Job drawing, mm, ordinate dimensions from the low corner. One solid piece. A direction names the side the tool comes from. Round coordinates to 2 decimals unless told otherwise and drop trailing zeros. Write each loop counter-clockwise with the first axis right and the second up, starting at its lowest first coordinate (ties: lowest second). Pieces come first, ordered by that corner, then holes. Notation, with made-up numbers: M 89,-6.75 L 110,-6.75 A35 cw 110,29.25 Z; hole C 16,63 d7. An arc over 180 degrees is marked long. Answer as a JSON object with one key per item and string values. Group by question number.
1. Which spindle directions (+Z, -Z, +X, -X, +Y, -Y) get a long thin tool onto all of the face, cutting with end or side? Do the marked faces 1, 2, 3, 4 and 5. Say none if no direction does.
2. Band-saw the part on D-D, the plane z = 2.5. Write the cut outline in (x, y).
3. Band-saw the part on B-B, the plane x = 10. Write the cut outline in (y, z) (1 decimal), plus the area to 3 significant figures.
4. Drop flat-ended pins along their axis: pin 1 (8 mm diameter, centred on y = 30.5, z = 3.5, fed in from +X); pin 2 (3 mm diameter, centred on x = 12, z = 3.5, fed in from -Y); pin 3 (6.5 mm diameter, centred on x = 18, z = 14.5, fed in from +Y); pin 4 (3 mm diameter, centred on x = 10, y = 10, fed in from +Z). Give the stop position or say it passes through.
5. Two-plate mould, pull along Y, no slides. Class the marked faces 6, 7, 8 and 9: +Y half, -Y half, draft (parallel to the pull), parting line (faces both ways), or undercut.
6. Band-saw the part on C-C, the plane x = 17. Write the cut outline in (y, z).
7. Drill centre lines: line 1 (Y direction, x = 10, z = 16.5) (1 decimal); line 2 (X direction, y = 37, z = 17.25); line 3 (Z direction, x = 16.75, y = 18). Where is each one in solid material? Low to high. Write a range as from..to.
8. Band-saw the part on A-A, the plane y = 10. Write the cut outline in (x, z) (1 decimal), plus the area to 3 significant figures.
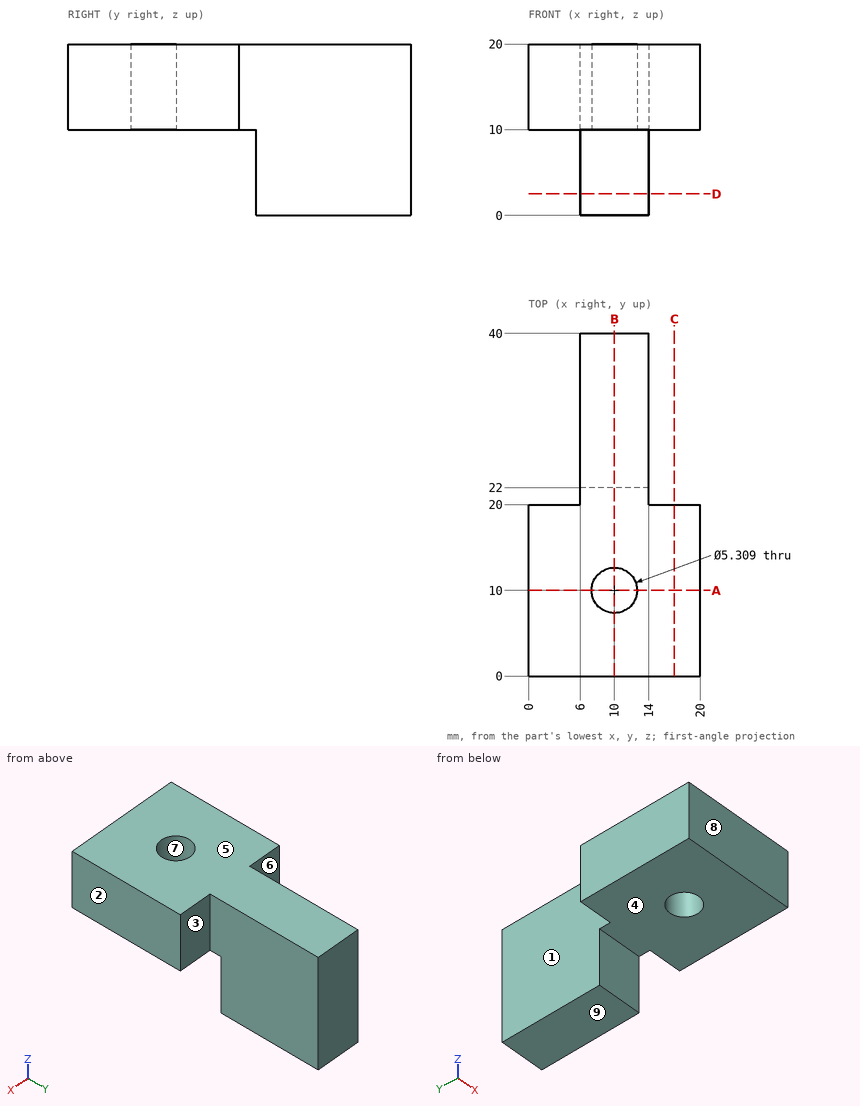
Worked answers:
{
 "1": {"face 1": "+Z, -Z, -X, +Y", "face 2": "+Z, -Z, +X, +Y, -Y", "face 3": "+Z, -Z, +X, +Y", "face 4": "-Z, +X, -X, -Y", "face 5": "+Z, +X, -X, +Y, -Y"},
 "2": {"outline": "M 6,22 L 14,22 L 14,40 L 6,40 Z"},
 "3": {"outline": "M 0,10 L 7.3,10 L 7.3,20 L 0,20 Z; M 12.7,10 L 22,10 L 22,0 L 40,0 L 40,20 L 12.7,20 Z", "area": "527 mm^2"},
 "4": {"pin 1": "stops at x = 14", "pin 2": "stops at y = 22", "pin 3": "stops at y = 20", "pin 4": "passes through"},
 "5": {"face 6": "+Y half", "face 7": "undercut", "face 8": "-Y half", "face 9": "draft"},
 "6": {"outline": "M 0,10 L 20,10 L 20,20 L 0,20 Z"},
 "7": {"line 1": "y = 0..7.3, 12.7..40", "line 2": "x = 6..14", "line 3": "z = 10..20"},
 "8": {"outline": "M 0,10 L 7.3,10 L 7.3,20 L 0,20 Z; M 12.7,10 L 20,10 L 20,20 L 12.7,20 Z", "area": "147 mm^2"}
}
